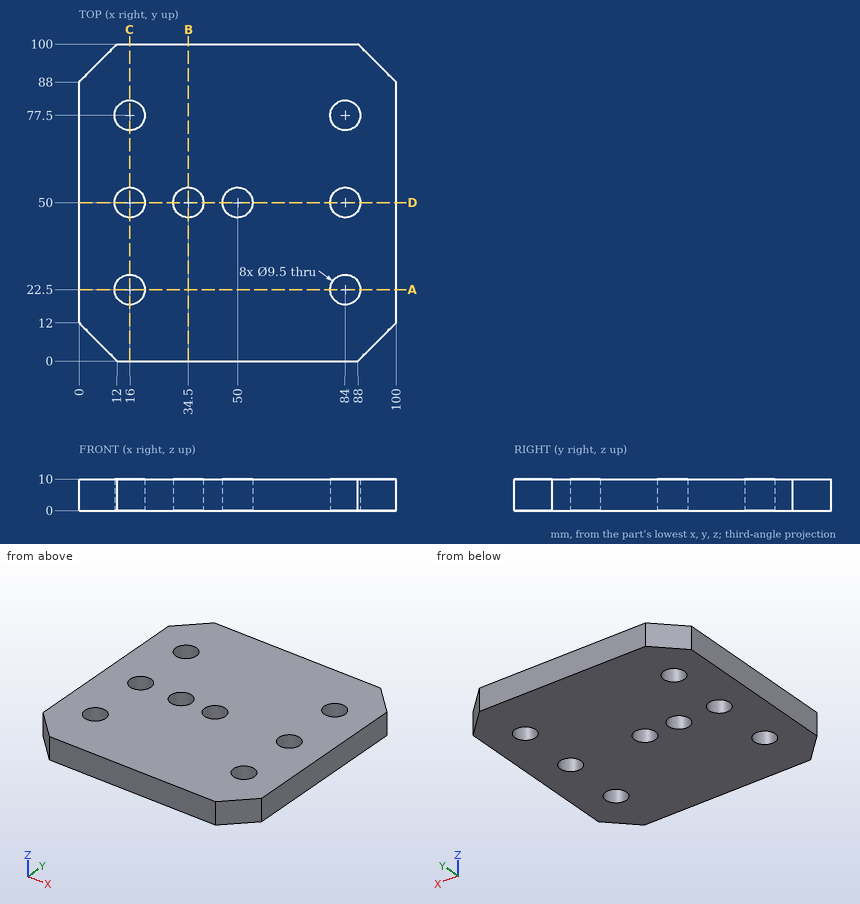
Check sheet for the drawn part. Datum: minimum x, y, z corner. Units: mm. Round coordinates to 2 decimals unless told otherwise and drop trailing zeros. Write each loop counter-clockwise with the first axis right and the second up, starting at its lowest first coordinate (ties: lowest second). Pieces come first, ordered by that corner, then holes. Notation, with made-up numbers: (-17.5, 87.25) -> (-8.5, 87.25) arc R25 cw to (-8.5, 121.25) -> close; hole circle Ø10 at (87, -34.75). An arc over 180 degrees is marked (long way). Put each result on its own line as item: value.
(1) Material ranges on line 1 (Y direction, x = 16, z = 6.5); line 2 (X direction, y = 23, z = 9.25); line 3 (Y direction, x = 13, z = 6.5), recorded low to high.
Values found:
line 1: y = 0 to 17.75, 27.25 to 45.25, 54.75 to 72.75, 82.25 to 100
line 2: x = 0 to 11.28, 20.72 to 79.28, 88.72 to 100
line 3: y = 0 to 18.82, 26.18 to 46.32, 53.68 to 73.82, 81.18 to 100
(2) Go/stop test with a flat-tipped pin: pin 1 Ø5.5 at (x, y) = (84, 22.5) entering from +Z. Record where the tip stops, or that it passes through.
Values found:
pin 1: passes through
(3) Sectioned sample at B-B (x = 34.5). Enter the section's corners in (y, z).
Values found:
outline: (0, 0) -> (45.25, 0) -> (45.25, 10) -> (0, 10) -> close; (54.75, 0) -> (100, 0) -> (100, 10) -> (54.75, 10) -> close
(4) Sectioned sample at D-D (y = 50). Enter the section's corners in (x, z).
Values found:
outline: (0, 0) -> (11.25, 0) -> (11.25, 10) -> (0, 10) -> close; (20.75, 0) -> (29.75, 0) -> (29.75, 10) -> (20.75, 10) -> close; (39.25, 0) -> (45.25, 0) -> (45.25, 10) -> (39.25, 10) -> close; (54.75, 0) -> (79.25, 0) -> (79.25, 10) -> (54.75, 10) -> close; (88.75, 0) -> (100, 0) -> (100, 10) -> (88.75, 10) -> close
(5) Sectioned sample at A-A (y = 22.5). Enter the section's corners in (x, z).
Values found:
outline: (0, 0) -> (11.25, 0) -> (11.25, 10) -> (0, 10) -> close; (20.75, 0) -> (79.25, 0) -> (79.25, 10) -> (20.75, 10) -> close; (88.75, 0) -> (100, 0) -> (100, 10) -> (88.75, 10) -> close
(6) Sectioned sample at C-C (x = 16). Enter the section's corners in (y, z), plus the area to 3 significant figures.
Values found:
outline: (0, 0) -> (17.75, 0) -> (17.75, 10) -> (0, 10) -> close; (27.25, 0) -> (45.25, 0) -> (45.25, 10) -> (27.25, 10) -> close; (54.75, 0) -> (72.75, 0) -> (72.75, 10) -> (54.75, 10) -> close; (82.25, 0) -> (100, 0) -> (100, 10) -> (82.25, 10) -> close
area: 715 mm^2
